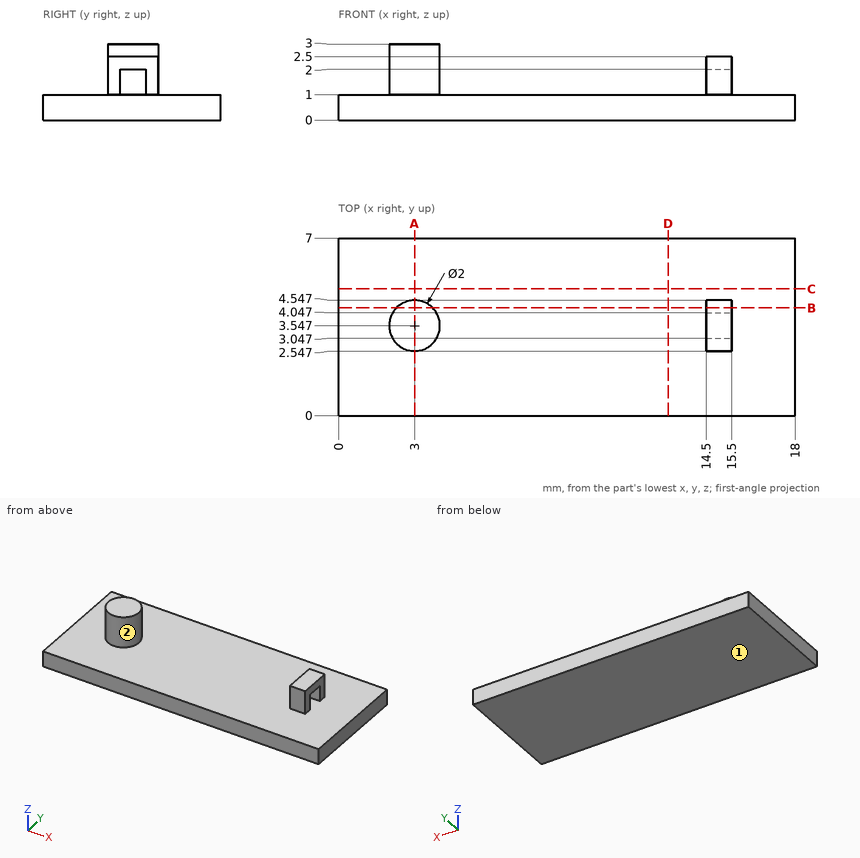
Answer from the drawing. Dimensions are ordinates in mm from the lowest x, y and z of the part. Give positions to 0.01 mm unless a question says otherwise; leave off trailing zeros. Write each loop counter-clockwise with the first axis right and the second up, starting at its lowest first coordinate (ties: lowest second). Pieces come first, ordered by that corner, then holes.
1) For a pull along X with two mould halves and no side action, classify the marked faces 1 and 2 as pulls with the +X half, pulls with the -X half, needs draft (parallel to the pull), parting line crosses it, or undercut.
2) Section D-D (x = 13) is taken. Write down the section's boundary in (y, z).
3) Section A-A (x = 3) is taken. Write down the section's boundary in (y, z), and give its area (3 significant figures).
4) Section B-B (y = 4.25) is taken. Write down the section's boundary in (x, z).
5) Given P1, Ø1.1, axis at x = 15, z = 2, coming from the +Y side; P2, Ø3.5, axis at x = 10, y = 2, coming from the +Z side, each flat-ended and moving along its own axis, determine where each tip first touches the part or whether it passes through.
6) Find the intervals of material crossed by L1, parallel to Z at x = 1.5, y = 2.25; L2, parallel to X at y = 3.5, z = 1.95; L3, parallel to X at y = 2.75, z = 1.45 (1 decimal), in increasing order.
7) Section C-C (y = 5) is taken. Write down the section's boundary in (x, z), and give its area (3 significant figures).
Response:
1. face 1: needs draft
1. face 2: undercut
2. outline: (0, 0) - (7, 0) - (7, 1) - (0, 1) - close
3. outline: (0, 0) - (7, 0) - (7, 1) - (4.55, 1) - (4.55, 3) - (2.55, 3) - (2.55, 1) - (0, 1) - close
3. area: 11.0 mm2
4. outline: (0, 0) - (18, 0) - (18, 1) - (15.5, 1) - (15.5, 2.5) - (14.5, 2.5) - (14.5, 1) - (3.71, 1) - (3.71, 3) - (2.29, 3) - (2.29, 1) - (0, 1) - close
5. P1: stops at y = 4.55
5. P2: stops at z = 1
6. L1: z = 0 to 1
6. L2: x = 2 to 4
6. L3: x = 2.4 to 3.6, 14.5 to 15.5
7. outline: (0, 0) - (18, 0) - (18, 1) - (0, 1) - close
7. area: 18.0 mm2
